The listing builds one solid part. Answer for the finished solid, in the listing's coordinates (mm). A direction names the side the tool comes from. Coordinates: 2 decimals unless noted, no trailing zeros. Order: outer loops, then holes, each group sorted by start corner. A loop starts at its lowest first (then second) coordinate and runs counter-clockwise, first axis right, second up.
Autodesk Inventor part; units mm, degrees
ref_plane "YZ Plane" through (0, 0, 0) normal (1, 0, 0) x (0, 1, 0)
ref_plane "XZ Plane" through (0, 0, 0) normal (0, 1, 0) x (-1, 0, 0)
ref_plane "XY Plane" through (0, 0, 0) normal (0, 0, 1) x (1, 0, 0)
sketch "Sketch1" plane through (0, 0, 0) normal (0, 1, 0) x (-1, 0, 0)
  line L0 (0, 0) -> (35, 0)
  line L1 (35, 0) -> (35, -43.79)
  line L2 (35, -43.79) -> (0, -43.79)
  line L3 (0, -43.79) -> (0, 0)
  dimension "d0" = 35
  dimension "d1" = 43.79
extrude "Extrusion1" add sketch "Sketch1" along normal blind 21.37
sketch "Sketch2" plane through (-35, 0, 0) normal (0, 0, 1) x (1, 0, 0)
  circle A0 centre (8.49, 10.185) radius 7.5
  circle A1 centre (25.49, 10.185) radius 7.5
  point P0 (35, 0)
  dimension "d4" = 15
  dimension "d5" = 15
extrude "Extrusion2" cut sketch "Sketch2" against normal blind 35.79
sketch "Sketch3" plane through (-35, 0, 0) normal (0, 0, 1) x (1, 0, 0)
  circle A0 centre (25.49, 10.185) radius 7.5
  circle A1 centre (25.49, 10.185) radius 8.5
  point P0 (35, 0)
  dimension "d9" = 17
extrude "Extrusion3" cut sketch "Sketch3" against normal blind 1.73
sketch "Sketch4" plane through (-35, 0, 0) normal (0, 0, 1) x (1, 0, 0)
  circle A0 centre (2.02, 19.35) radius 1.02
  circle A1 centre (33.17, 2.02) radius 1.02
  point P0 (35, 0)
  dimension "d12" = 2.04
  dimension "d13" = 2.04
extrude "Extrusion4" cut sketch "Sketch4" against normal blind 2.1
sketch "Sketch5" plane through (0, 0, 0) normal (0, -1, 0) x (1, 0, 0)
  circle A0 centre (-32.19, -3) radius 1.02
  circle A1 centre (-3, -40.79) radius 1.02
  point P0 (0, 0)
  dimension "d17" = 2.04
  dimension "d23" = 2.04
extrude "Extrusion5" cut sketch "Sketch5" against normal blind 2.1
sketch "Sketch6" plane through (0, 0, 0) normal (0, -1, 0) x (1, 0, 0)
  circle A0 centre (-18.19, -15.39) radius 1.02
  circle A1 centre (-18.19, -31.79) radius 1.02
  point P0 (0, 0)
  dimension "d20" = 2.04
  dimension "d21" = 2.04
extrude "Extrusion6" cut sketch "Sketch6" against normal blind 6.1
sketch "Sketch10" plane through (0, 21.37, 0) normal (0, 1, 0) x (1, 0, 0)
  line L0 (-35, 43.79) -> (-35, 0)
  line L1 (0, 0) -> (0, 43.79)
  line L2 (-35, 43.79) -> (0, 43.79)
  line L3 (0, 43.79) -> (0, 3.79)
  line L4 (0, 3.79) -> (-35, 3.79)
  line L5 (-35, 3.79) -> (-35, 43.79)
  line L6 (-34, 4.79) -> (-1, 4.79)
  line L7 (-1, 4.79) -> (-1, 42.79)
  line L8 (-1, 42.79) -> (-34, 42.79)
  line L9 (-34, 42.79) -> (-34, 4.79)
  dimension "d30" = 40
  dimension "d31" = 1
extrude "Extrusion8" cut sketch "Sketch10" against normal blind 2 contours L9 L8 L7 L6
sketch "Sketch11" plane through (-35, 0, 0) normal (0, 0, 1) x (1, 0, 0)
  line L0 (35, 21.37) -> (0, 21.37)
  circle A0 centre (31.7551, 21.37) radius 2.79
  point P0 (35, 0)
  dimension "d34" = 5.58
extrude "Extrusion9" cut sketch "Sketch11" against normal through all
sketch "Sketch12" plane through (0, 19.37, 0) normal (0, 1, 0) x (1, 0, 0)
  line L0 (-34, 4.79) -> (-34, 42.79)
  line L1 (-5.1902, 4.79) -> (-5.1902, 42.79)
  line L2 (-34, 42.79) -> (-5.1902, 42.79)
  line L3 (-5.1902, 42.79) -> (-5.1902, 4.79)
  line L4 (-5.1902, 4.79) -> (-34, 4.79)
  line L5 (-34, 4.79) -> (-34, 42.79)
  line L6 (-33, 5.79) -> (-6.1902, 5.79)
  line L7 (-6.1902, 5.79) -> (-6.1902, 41.79)
  line L8 (-6.1902, 41.79) -> (-33, 41.79)
  line L9 (-33, 41.79) -> (-33, 5.79)
  point P0 (0, 0)
  dimension "d37" = 1
extrude "Extrusion10" add sketch "Sketch12" along normal blind 1 contours L9 L8 L7 L6
properties part number "Small LRF Real"
1) Each of these flat-tipped pins is pushed along its axis until it touches: P1, Ø1.2, axis at x = -3, z = -40.79, coming from the -Y side; P2, Ø0.6, axis at x = -18.5, z = -31.5, coming from the -Y side; P3, Ø4, axis at x = -9, z = -27.5, coming from the +Y side. Where does it stop, or does it pass through?
2) Consider L1, parallel to X at y = 20, z = -32; L2, parallel to X at y = 8, z = -31.5; L3, parallel to Z at x = -32.19, y = 1.75. Determine where each line is inside the solid, lowest interval first.
3) Section B-B (y = 13.5) is taken. Give the vertices of the cut face in (x, z).
4) Section A-A (z = -40.79) is taken. Give the vertices of the cut face in (x, y), then the cut area to 3 significant figures.
5) Section D-D (x = -15) is taken. Give the vertices of the cut face in (y, z).
6) Section C-C (z = -15.39) is taken. Give the vertices of the cut face in (x, y) (3 decimals).
7) Determine the mould class of faces 6 (the face through (-17.3, 5.8, 0)), 7 (the face through (-35, 11, -22)), 8 (the face through (-18, 6.1, -32)) for opening direction Z: released by +Z, released by -Z, zero draft, split by the parting line, or undercut.
8) A tool of negligible diameter and unlimited length cuts with its end or side. For faces 1 (the face through (-23, 21.37, -4)), 2 (the face through (-2.349, 18.728, -21.588)), 3 (the face through (-19, 20, -42.79)), 4 (the face through (-1.28, 2.88, -1.04)), 5 (the face through (-31.248, 1.035, -3.391)), from which of +Z, -Z, +X, -X, +Y, -Y can it reach the whole face along a straight path? Write none if from no direction.
Filled sheet:
1. P1: stops at y = 2.1
1. P2: stops at y = 6.1
1. P3: stops at y = 20.37
2. L1: x = -35 to -34, -33 to -6.19, -0.81 to 0
2. L2: x = -35 to -33.68, -19.34 to -16.68, -2.34 to 0
2. L3: z = -43.79 to -4.02, -1.98 to 0
3. outline: (-35, -43.79) - (0, -43.79) - (0, 0) - (-1.68, 0) - (-1.68, -1.73) - (-2.78, -1.73) - (-2.78, -35.79) - (-16.24, -35.79) - (-16.24, -1.73) - (-17.34, -1.73) - (-17.34, 0) - (-19.78, 0) - (-19.78, -35.79) - (-33.24, -35.79) - (-33.24, 0) - (-35, 0) - close
4. outline: (-35, 0) - (-4.02, 0) - (-4.02, 2.1) - (-1.98, 2.1) - (-1.98, 0) - (0, 0) - (0, 21.37) - (-0.45, 21.37) arc R2.79 cw to (-1, 19.71) - (-1, 19.37) - (-1.3, 19.37) arc R2.79 cw to (-5.19, 19.37) - (-6.19, 19.37) - (-6.19, 20.37) - (-33, 20.37) - (-33, 19.37) - (-34, 19.37) - (-34, 21.37) - (-35, 21.37) - close
4. area: 702 mm2
5. outline: (0, -43.79) - (21.37, -43.79) - (21.37, -42.79) - (19.37, -42.79) - (19.37, -41.79) - (20.37, -41.79) - (20.37, -5.79) - (19.37, -5.79) - (19.37, -4.79) - (21.37, -4.79) - (21.37, 0) - (16.67, 0) - (16.67, -1.73) - (15.29, -1.73) - (15.29, -35.79) - (5.08, -35.79) - (5.08, -1.73) - (3.7, -1.73) - (3.7, 0) - (0, 0) - close
6. outline: (-35, 0) - (-19.21, 0) - (-19.21, 6.1) - (-17.17, 6.1) - (-17.17, 0) - (0, 0) - (0, 21.37) - (-0.455, 21.37) arc R2.79 cw to (-1, 19.713) - (-1, 19.37) - (-1.3, 19.37) arc R2.79 cw to (-5.19, 19.37) - (-6.19, 19.37) - (-6.19, 20.37) - (-33, 20.37) - (-33, 19.37) - (-34, 19.37) - (-34, 21.37) - (-35, 21.37) - close; hole circle Ø15 at (-26.51, 10.185); hole circle Ø15 at (-9.51, 10.185)
7. face 6: released by +Z
7. face 7: zero draft
7. face 8: undercut
8. face 1: +Z, -Z, +X, -X, +Y
8. face 2: +Z, -Z, +Y
8. face 3: +Y
8. face 4: +Z
8. face 5: -Y
